Autodesk Inventor part; units mm, degrees
ref_plane "YZ Plane" through (0, 0, 0) normal (1, 0, 0) x (0, 1, 0)
ref_plane "XZ Plane" through (0, 0, 0) normal (0, 1, 0) x (-1, 0, 0)
ref_plane "XY Plane" through (0, 0, 0) normal (0, 0, 1) x (1, 0, 0)
sketch "Sketch1" plane through (0, 0, 0) normal (0, 0, 1) x (1, 0, 0)
  line L0 (3, -25) -> (44.33, -25)
  line L1 (44.33, -25) -> (44.33, -28)
  line L2 (44.33, -28) -> (35, -28)
  line L3 (35, -28) -> (3, -45)
  line L4 (3, -45) -> (3, -56.285)
  line L5 (3, -56.285) -> (0, -56.285)
  line L6 (0, -56.285) -> (0, 0)
  line L7 (3, -41.6029) -> (28.6055, -28)
  line L8 (28.6055, -28) -> (3, -28)
  line L9 (3, -41.6029) -> (3, -28)
  line L10 (0, -4.33) -> (3, -4.33) construction
  line L11 (0, -2.08) -> (3, -2.08) construction
  line L12 (0, -6.58) -> (3, -6.58) construction
  line L13 (0, -51.955) -> (3, -51.955) construction
  line L14 (0, -49.705) -> (3, -49.705) construction
  line L15 (0, -54.205) -> (3, -54.205) construction
  line L16 (40, -25) -> (40, -28) construction
  line L17 (0, 0) -> (3, 0)
  line L18 (3, 0) -> (3, -25)
  dimension "d1" = 3
  dimension "d2" = 3
  dimension "d3" = 3
  dimension "d6" = 20
  dimension "d8" = 4.5
  dimension "d13" = 47.625
  dimension "d18" = 40
  dimension "d48" = 4.33
  dimension "d49" = 5
  dimension "d55" = 4.33
  dimension "d56" = 25
  dimension "d59" = 4.33
extrude "Extrusion1" add sketch "Sketch1" along normal mid plane 10
fillet "Fillet2" radius 2 6 edges at (3, -45, 0) (35, -28, 0) (28.6055, -28, 0) (3, -41.6029, 0) (3, -28, 0) (3, -25, 0)
sketch "Sketch3" plane through (0, -56.285, 5) normal (-1, 0, 0) x (0, 0, 1)
  line L0 (-2.4019, 51.955) -> (-3.701, 49.705)
  line L1 (-3.701, 49.705) -> (-6.299, 49.705)
  line L2 (-6.299, 49.705) -> (-7.5981, 51.955)
  line L3 (-7.5981, 51.955) -> (-6.299, 54.205)
  line L4 (-6.299, 54.205) -> (-3.701, 54.205)
  line L5 (-3.701, 54.205) -> (-2.4019, 51.955)
  line L6 (-6.299, 6.58) -> (-3.701, 6.58)
  line L7 (-3.701, 6.58) -> (-2.4019, 4.33)
  line L8 (-2.4019, 4.33) -> (-3.701, 2.08)
  line L9 (-3.701, 2.08) -> (-6.299, 2.08)
  line L10 (-6.299, 2.08) -> (-7.5981, 4.33)
  line L11 (-7.5981, 4.33) -> (-6.299, 6.58)
  point P0 (-5, 56.285)
  point P1 (-5, 51.955)
  point P2 (-5, 51.955)
  point P3 (-5, 4.33)
  point P4 (-5, 4.33)
  dimension "d60" = 4.5
extrude "Extrusion3" cut sketch "Sketch3" against normal through all
sketch "Sketch4" plane through (44.33, -25, 5) normal (0, 1, 0) x (1, 0, 0)
  line L0 (-39.33, 10) -> (0, 10) construction
  line L1 (-4.33, 10) -> (0.0001, 7.5)
  line L2 (0.0001, 7.5) -> (0.0001, 2.5)
  line L3 (0.0001, 2.5) -> (-4.33, 0)
  line L4 (-4.33, 0) -> (-8.6601, 2.5)
  line L5 (-8.6601, 2.5) -> (-8.6601, 7.5)
  line L6 (-8.6601, 7.5) -> (-4.33, 10)
  line L7 (-4.33, 6.9053) -> (-2.68, 5.9526)
  line L8 (-2.68, 5.9526) -> (-2.68, 4.0474)
  line L9 (-2.68, 4.0474) -> (-4.33, 3.0947)
  line L10 (-4.33, 3.0947) -> (-5.98, 4.0474)
  line L11 (-5.98, 4.0474) -> (-5.98, 5.9526)
  line L12 (-5.98, 5.9526) -> (-4.33, 6.9053)
  point P0 (-44.33, 5)
  point P1 (-4.33, 5)
  point P2 (-4.33, 5)
  point P3 (-4.33, 5)
  dimension "d63" = 3.3
extrude "Extrusion4" add sketch "Sketch4" along normal blind 2
extrude "Extrusion5" cut sketch "Sketch4" against normal through all contours L7 L8 L9 L10 L11 L12
chamfer "Chamfer1" distance 2.5 angle 60 2 edges at (44.33, -26.5, 5) (44.33, -26.5, -5) measured on face at (44.33, -27, -0.8334)
chamfer "Chamfer2" distance 2.5 angle 60 2 edges at (1.5, 0, -5) (1.5, 0, 5) measured on face at (2, 0, -1.6667)
chamfer "Chamfer3" distance 2.5 angle 60 2 edges at (1.5, -56.285, 5) (1.5, -56.285, -5) measured on face at (2, -56.285, 1.6667)
properties part number "GPS_holder"
Can you work these out from the model? Positions are in its coordinate system, mm. A direction names the side the tool comes from. Round coordinates to 2 decimals unless told otherwise and drop trailing zeros. Order: outer loops, then holes, each group sorted by start corner. A loop starts at its lowest first (then second) coordinate and runs counter-clockwise, first axis right, second up.
(1) If we section it at B-B (x = 9): Please give me the cut outline in (y, z), plus the area to 3 significant figures.
Results are:
outline: (-41.81, -5) - (-38.42, -5) - (-38.42, 5) - (-41.81, 5) - close; (-28, -5) - (-25, -5) - (-25, 5) - (-28, 5) - close
area: 64.0 mm2
(2) If I drill on L1, parallel to Y at x = 2, z = -1.5 (3 decimals); L2, parallel to X at y = -17, z = 4.75; L3, parallel to Y at x = 11, z = -1, over which ranges is the centre line in solid material (lowest first)?
Results are:
L1: y = -56.285 to -53.857, -50.053 to -6.232, -2.428 to 0
L2: x = 0 to 3
L3: y = -40.75 to -37.35, -28 to -25
(3) If we section it at C-C (y = -35): Please give me the cut outline in (x, z), plus the area to 3 significant figures.
Results are:
outline: (0, -5) - (3, -5) - (3, 5) - (0, 5) - close; (15.43, -5) - (21.82, -5) - (21.82, 5) - (15.43, 5) - close
area: 93.9 mm2
(4) We'd pull the mould along Y, two halves only. Please class faces 1 (the face through (3.945, -39.975, 0.07)), 2 (the face through (1.52, -2.2, -3.77)), 3 (the face through (11, -26, 5)): +Y half, -Y half, draft (parallel to the pull), parting line (faces both ways), or undercut.
Results are:
face 1: undercut
face 2: +Y half
face 3: draft
(5) On a 3-axis mill with a long thin cutter (end or side, diameter ignored), from which of +Z, -Z, +X, -X, +Y, -Y can I reach the whole of each face in a straight line? I mean faces 4 (the face through (1, -54.205, 0)), 5 (the face through (40.84, -25.54, 1.42)), 6 (the face through (3, -49, 0)), 7 (the face through (39.9, -23, 2.2)), 8 (the face through (13.62, -35.96, -0.07)). Say none if no direction works.
Results are:
face 4: +X, -X
face 5: +Y, -Y
face 6: +Z, -Z, +X, -Y
face 7: +Z, -Z, +X, +Y
face 8: +Z, -Z
(6) I'm going to push flat-ended pins straight in: pin 1 (4 mm diameter, centred on y = -13.5, z = 2.5, fed in from +X); pin 2 (4 mm diameter, centred on x = 7, z = 0, fed in from +Y); pin 3 (5 mm diameter, centred on x = 9, z = 0, fed in from -Y). Where does each tip first touch, or does it pass through?
Results are:
pin 1: stops at x = 3
pin 2: stops at y = -25
pin 3: stops at y = -43.14
(7) If we section it at A-A (z = -0.25): Count the separate pieces of the cut face and the enclosed holes in it, plus the area to 3 significant figures.
Results are:
separate pieces: 4
enclosed holes: 1
area: 380 mm2
